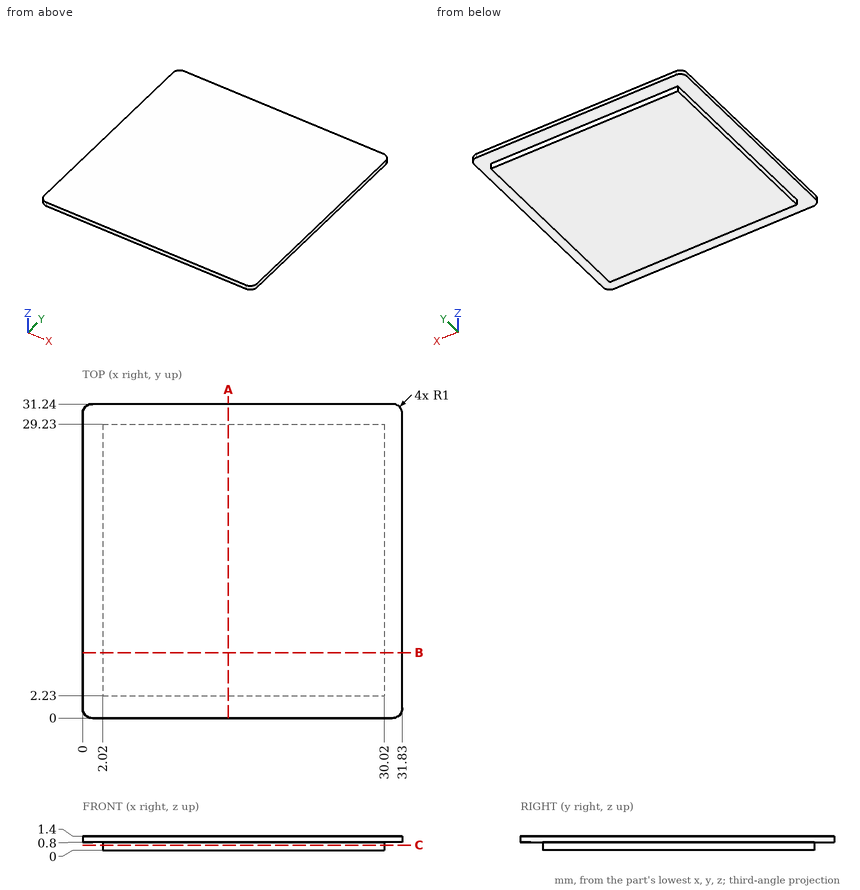
Design review of the part shown in the three views and the two pictorial views. Dimensions are in mm from the part's minimum x, y and z. Give positions to 0.01 mm unless a question says otherwise; leave off trailing zeros. Write each loop counter-clockwise with the first axis right and the second up, starting at its lowest first coordinate (ties: lowest second). Pieces come first, ordered by that corner, then holes.
Item 1: Take a section at B-B (y = 6.5). Give the boundary of the cut face in (x, z).
Item 2: Take a section at C-C (z = 0.5). Give the boundary of the cut face in (x, y), and give its area (3 significant figures).
Item 3: Take a section at A-A (x = 14.5). Give the boundary of the cut face in (y, z).
Item 4: Wall thickness on probe 1 along X at (y, z) = (24.5, 0.3); probe 2 along Y at (x, z) = (3, 0.55); probe 3 along Z at (x, y) = (17, 2): over which ranges is each line inside the solid? List them lowest first.
Established:
1. outline: (0, 0.8) - (2.02, 0.8) - (2.02, 0) - (30.02, 0) - (30.02, 0.8) - (31.83, 0.8) - (31.83, 1.4) - (0, 1.4) - close
2. outline: (2.02, 2.23) - (30.02, 2.23) - (30.02, 29.23) - (2.02, 29.23) - close
2. area: 756 mm2
3. outline: (0, 0.8) - (2.23, 0.8) - (2.23, 0) - (29.23, 0) - (29.23, 0.8) - (31.24, 0.8) - (31.24, 1.4) - (0, 1.4) - close
4. probe 1: x = 2.02 to 30.02
4. probe 2: y = 2.23 to 29.23
4. probe 3: z = 0.8 to 1.4
